Here's how the part is built. I have some questions about the finished solid (model axes, mm). A direction names the side the tool comes from. Round coordinates to 2 decimals unless told otherwise and drop trailing zeros. Loops run counter-clockwise (first coordinate to the right, second up) from the corner with the lowest first, then second, coordinate; pieces in that order, holes last. Notation, with made-up numbers: M -34,32 L -18,32 A13 cw -18,36 Z; hole C 55,66.5 d5. An arc over 180 degrees is marked long. Use a Markdown table: item, result.
from build123d import *

# Parameters (mm, degrees)
ESQUISSE1_W             = 24
ESQUISSE1_H             = 80
BOSS_EXTRU_1_DEPTH      = 4
ESQUISSE2_W             = 24
ESQUISSE2_H             = 23
BOSS_EXTRU_2_DEPTH      = 4
BOSS_EXTRU_3_DEPTH      = 16
ESQUISSE4_W             = 6
ESQUISSE4_H             = 37
BOSS_EXTRU_4_DEPTH      = 4
CHANFREIN1_SIZE         = 4
CHANFREIN2_SIZE2        = 4.617363823
CHANFREIN2_SIZE         = 20
D_GAGEMENT_M31_D        = 3.4
D_GAGEMENT_M42_D        = 4.3
ESQUISSE11_R            = 3.2
ENL_V_MAT_EXTRU_1_DEPTH = 3


with BuildPart() as part:
    # Esquisse1 → Boss.-Extru.1 (new body)
    with BuildSketch(Plane.XY):
        Rectangle(ESQUISSE1_W, ESQUISSE1_H)
    extrude(amount=BOSS_EXTRU_1_DEPTH)

    # Esquisse2 → Boss.-Extru.2 (add)
    with BuildSketch(Plane.XY.offset(4)):
        with Locations((0, 8.5)):
            Rectangle(ESQUISSE2_W, ESQUISSE2_H)
    extrude(amount=BOSS_EXTRU_2_DEPTH)

    # Esquisse3 → Boss.-Extru.3 (add)
    with BuildSketch(Plane.XY.offset(8)):
        Polygon((-6, 20), (-6, 0), (6, 0), (6, 20), (12, 20), (12, -3), (-12, -3), (-12, 20), align=None)
    extrude(amount=BOSS_EXTRU_3_DEPTH)

    # Esquisse4 → Boss.-Extru.4 (add)
    with BuildSketch(Plane.XY.offset(4)):
        with Locations((-9, -21.5)):
            Rectangle(ESQUISSE4_W, ESQUISSE4_H)
        with Locations((9, -21.5)):
            Rectangle(ESQUISSE4_W, ESQUISSE4_H)
    extrude(amount=BOSS_EXTRU_4_DEPTH)

    # Chanfrein1
    chanfrein1_edges = [part.edges().sort_by_distance(p)[0] for p in [
        (-9, -40, 8),
        (9, -40, 8),
        (12, 40, 2),
        (-12, 40, 2),
    ]]
    chamfer(chanfrein1_edges, length=CHANFREIN1_SIZE)

    # Chanfrein2
    chanfrein2_edges = [part.edges().sort_by_distance(p)[0] for p in [
        (-9, 20, 24),
    ]]
    chanfrein2_side = [part.faces().sort_by_distance(p)[0] for p in [
        (-9, 20, 23.907652724),
    ]]
    chamfer(chanfrein2_edges, length=CHANFREIN2_SIZE - 0.0001, length2=CHANFREIN2_SIZE2 - 0.0001, reference=chanfrein2_side[0])  # a hair under: the kernel refuses the full size

    # Dégagement M31 (through all)
    with Locations(Plane(origin=(12, 0, 0), x_dir=(0, 0, -1), z_dir=(1, 0, 0))):
        with Locations((-18, 10)):
            Hole(D_GAGEMENT_M31_D / 2)

    # Dégagement M42 (through all)
    with Locations(Plane.XY.offset(4)):
        with Locations((0, 30), (0, -30)):
            Hole(D_GAGEMENT_M42_D / 2)

    # Esquisse11 → Enlèv. mat.-Extru.1 (cut)
    with BuildSketch(Plane.ZY.offset(12)):
        with Locations(Location((18, 10, 0), (0, 0, 270))):
            Circle(ESQUISSE11_R)
    extrude(amount=-ENL_V_MAT_EXTRU_1_DEPTH, mode=Mode.SUBTRACT)


solid = part.part
1. Which directions (+Z, -Z, +X, -X, +Y, -Y) give clear straight access to the entire face, cutting with the end or side of a thin tool? Please do faces 5 (the face through (0, 0, 16)), 6 (the face through (-0.2, 32.4, 4)), 7 (the face through (-9, 8.6, 16.6)).
Answer sheet:
| item | result |
|---|---|
| face 5 | +Z, +Y |
| face 6 | +Z, +X, -X, +Y |
| face 7 | -X |
2. Imagine slicing it at A-A, the plane y = 10. Write out the boundary of the cut face in (x, z).
Answer sheet:
| item | result |
|---|---|
| outline | M -12,0 L 12,0 L 12,16.3 L 6,16.3 L 6,8 L -6,8 L -6,16.3 L -9,16.3 L -9,14.8 L -12,14.8 Z; M -12,21.2 L -9,21.2 L -9,19.7 L -6,19.7 L -6,24 L -12,24 Z; M 6,19.7 L 12,19.7 L 12,24 L 6,24 Z |
3. Imagine slicing it at B-B, the plane z = 3.25. Write out the boundary of the cut face in (x, y).
Answer sheet:
| item | result |
|---|---|
| outline | M -12,-40 L 12,-40 L 12,36 L 8,40 L -8,40 L -12,36 Z; hole C 0,-30 d4.3; hole C 0,30 d4.3 |
4. Imagine slicing it at D-D, the plane y = -30. Write out the boundary of the cut face in (x, z).
Answer sheet:
| item | result |
|---|---|
| outline | M -12,0 L -2.15,0 L -2.15,4 L -6,4 L -6,8 L -12,8 Z; M 2.15,0 L 12,0 L 12,8 L 6,8 L 6,4 L 2.15,4 Z |
5. Imagine slicing it at C-C, the plane x = 0. State how many separate pieces and enclosed holes the cut face has, then the cut area to 3 significant figures.
Answer sheet:
| item | result |
|---|---|
| separate pieces | 3 |
| enclosed holes | 0 |
| area | 424 mm2 |
6. I need wall thicknesses on probe 1 along Y at (x, z) = (0, 1.1); probe 2 along X at (y, z) = (-11, 4.5); probe 3 along Z at (x, y) = (-9.7, 10). Which ranges of each line are inside material? Lowest first, please. Write a range as from..to.
Answer sheet:
| item | result |
|---|---|
| probe 1 | -40..-32.15, -27.85..27.85, 32.15..40 |
| probe 2 | -12..-6, 6..12 |
| probe 3 | 0..14.8, 21.2..24 |
7. For pin 1 Ø3 at (y, z) = (9.5, 18) entering from -X; pin 2 Ø3 at (x, y) = (1.5, 8.5) entering from -Z; pin 3 Ø6.5 at (x, y) = (-10.5, -22.5) entering from +Z; pin 4 Ø2.5 at (y, z) = (10, 18) entering from -X, each with a flat end and sliding along its axis, tell me the tip position at first contact or that it passes through.
Answer sheet:
| item | result |
|---|---|
| pin 1 | x = -9 |
| pin 2 | z = 0 |
| pin 3 | z = 8 |
| pin 4 | through |
8. We'd pull the mould along Z, two halves only. Please class faces 1 (the face through (8.96, 9.35, 19.57)), 2 (the face through (0, 1, 0)), 3 (the face through (-10, 38, 2)), 4 (the face through (-9, -38, 6)): +Z half, -Z half, draft (parallel to the pull), parting line (faces both ways), or undercut.
Answer sheet:
| item | result |
|---|---|
| face 1 | undercut |
| face 2 | -Z half |
| face 3 | draft |
| face 4 | +Z half |
